Part model, mm, in its own coordinate system. Face numbers are marked on the shaded views. Give positions to 0.01 mm unless a question says otherwise; leave off trailing zeros. Write each loop counter-clockwise with the first axis right and the second up, starting at its lowest first coordinate (ties: lowest second). Pieces come first, ordered by that corner, then holes.
from build123d import *

# Parameters (mm, degrees)
F0_W     = 41.275
F0_H     = 15.875
F1_DEPTH = 19.05
F3_D     = 7.9375
F5_D     = 6.35


with BuildPart() as f1:
    # F0 (on Top) → F1 (new body)
    with BuildSketch(Plane.XY):
        with Locations((20.6375, 7.9375)):
            Rectangle(F0_W, F0_H)
    extrude(amount=F1_DEPTH)

    # F3 (through all)
    with Locations(Plane.XY.offset(19.05)):
        with Locations((20.6375, 7.9375)):
            Hole(F3_D / 2)

    # F5 (through all)
    with Locations(Plane.XZ):
        with Locations((6.35, 9.525), (34.925, 9.525)):
            Hole(F5_D / 2)


solid = f1.part
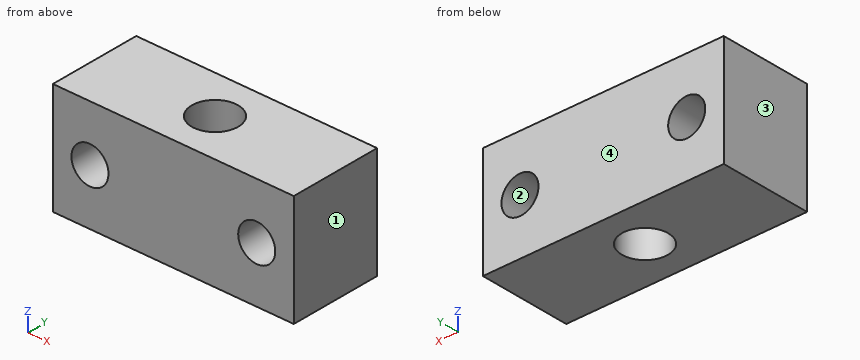
1) Saw through at D-D (z = 3.5). Write the cut outline in (x, y) (1 decimal).
Check result:
outline: (0, 0) - (41.3, 0) - (41.3, 15.9) - (0, 15.9) - close; hole circle Ø7.9 at (20.6, 7.9)
2) Mould opens along X. For the marked faces 1, 2, 3 and 4 say: +X half, -X half, draft (parallel to the pull), parting line (faces both ways), or undercut.
Check result:
face 1: +X half
face 2: undercut
face 3: -X half
face 4: draft
3) Flat gauge pin, fed straight in: P1, Ø6, axis at x = 15, z = 4.5, coming from the -Y side. Where does the tip first touch, or does it go through?
Check result:
P1: stops at y = 0
4) Saw through at C-C (y = 11.5). Write the cut outline in (x, z) (3 decimals).
Check result:
outline: (0, 0) - (18.888, 0) - (18.888, 19.05) - (0, 19.05) - close; (22.387, 0) - (41.275, 0) - (41.275, 19.05) - (22.387, 19.05) - close; hole circle Ø6.35 at (6.35, 9.525); hole circle Ø6.35 at (34.925, 9.525)
5) Saw through at A-A (z = 10.75). Write the cut outline in (x, y) (1 decimal).
Check result:
outline: (0, 0) - (3.4, 0) - (3.4, 15.9) - (0, 15.9) - close; (9.3, 0) - (32, 0) - (32, 15.9) - (9.3, 15.9) - close; (37.9, 0) - (41.3, 0) - (41.3, 15.9) - (37.9, 15.9) - close; hole circle Ø7.9 at (20.6, 7.9)
6) Drill centre lines: L1, parallel to X at y = 8, z = 5.5 (3 decimals); L2, parallel to X at y = 14, z = 9 (3 decimals); L3, parallel to X at y = 6.75, z = 8.75 (3 decimals). Where is each one in solid material? Low to high.
Check result:
L1: x = 0 to 16.669, 24.606 to 41.275
L2: x = 0 to 3.219, 9.481 to 31.794, 38.056 to 41.275
L3: x = 0 to 3.271, 9.429 to 16.851, 24.424 to 31.846, 38.004 to 41.275
7) Saw through at B-B (x = 6.35). Write the cut outline in (y, z) (3 decimals).
Check result:
outline: (0, 0) - (15.875, 0) - (15.875, 6.35) - (0, 6.35) - close; (0, 12.7) - (15.875, 12.7) - (15.875, 19.05) - (0, 19.05) - close
